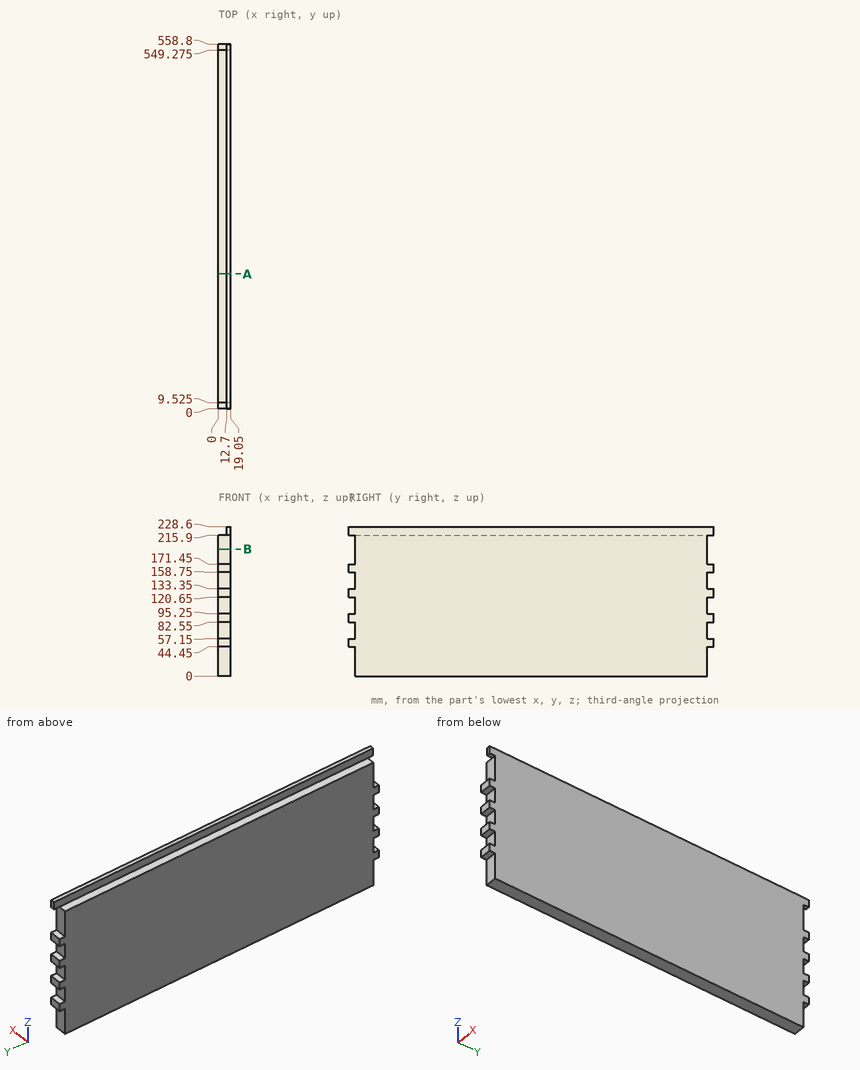
Could you check a few things on this drawing? It's one solid part, dimensions in mm from its lowest x, y, z. Round coordinates to 2 decimals unless told otherwise and drop trailing zeros. Loops run counter-clockwise (first coordinate to the right, second up) from the corner with the lowest first, then second, coordinate; pieces in that order, holes last. Notation, with made-up numbers: (-19.75, 0) -> (9.25, 0) arc R21 ccw to (9.25, 20) -> close; hole circle Ø7 at (-3, 25). An arc over 180 degrees is marked (long way). One line per item, written item: value. Start each with the question number.
1. If I drill on probe 1 along Z at (x, y) = (9.75, 232); probe 2 along Y at (x, z) = (6.25, 32) (3 decimals), over which ranges is the centre line in solid material (lowest first)?
2. For pin 1 (3 mm diameter, centred on x = 17, y = 552.5, fed in from -Z); pin 2 (9.5 mm diameter, centred on x = 6, z = 199, fed in from -Y) (3 decimals); pin 3 (9.5 mm diameter, centred on x = 6, z = 73.5, fed in from +Y) (3 decimals), each with a flat end and sliding along its axis, tell me the tip position at first contact or that it passes through.
3. If we section it at B-B, the plane z = 194.5: Write out the boundary of the cut face in (x, y) (3 decimals), then the cut area to 3 significant figures.
4. If we section it at A-A, the plane y = 206.5: Write out the boundary of the cut face in (x, z), then the cut area to 3 significant figures.
Calculated:
1. probe 1: z = 0 to 215.9
1. probe 2: y = 9.525 to 549.275
2. pin 1: stops at z = 44.45
2. pin 2: stops at y = 9.525
2. pin 3: stops at y = 549.275
3. outline: (0, 9.525) -> (19.05, 9.525) -> (19.05, 549.275) -> (0, 549.275) -> close
3. area: 10,300 mm²
4. outline: (0, 0) -> (19.05, 0) -> (19.05, 228.6) -> (12.7, 228.6) -> (12.7, 215.9) -> (0, 215.9) -> close
4. area: 4,190 mm²
